The listing builds one solid part. Answer for the finished solid, in the listing's coordinates (mm). A direction names the side the tool comes from. Give positions to 0.01 mm unless a question says otherwise; leave off trailing zeros. Write each loop counter-clockwise with the first axis right and the second up, starting at its lowest first coordinate (ties: lowest second). Pieces come first, ordered by that corner, then holes. Notation, with made-up numbers: M 17,47 L 70,47 A35 ccw 70,86 Z; hole C 78,75 d3. An arc over 180 degrees is marked long. Answer as a JSON object with one key per item and string values.
```python
from build123d import *

# Parameters (mm, degrees)
SKETCH_W      = 135
SKETCH_H      = 117
SKETCH_R      = 1.75
PAD_DEPTH     = 5
SKETCH001_W   = 36
SKETCH001_H   = 19.7
PAD001_DEPTH  = 4.8
SKETCH002_W   = 6
SKETCH002_H   = 28
SKETCH002_R   = 1.5
PAD002_DEPTH  = 4
SKETCH003_W   = 6
SKETCH003_H   = 28
SKETCH003_R   = 1.5
PAD003_DEPTH  = 4
SKETCH004_W   = 6
SKETCH004_H   = 28
SKETCH004_R   = 1.5
PAD004_DEPTH  = 4
SKETCH005_W   = 6
SKETCH005_H   = 28
SKETCH005_R   = 1.5
PAD005_DEPTH  = 4
SKETCH006_R   = 2.5
SKETCH006_R_2 = 1.65
PAD006_DEPTH  = 5
SKETCH007_W   = 4
SKETCH007_H   = 20
PAD007_DEPTH  = 8
SKETCH009_W   = 6
SKETCH009_H   = 6
SKETCH009_R   = 1.5
PAD009_DEPTH  = 32
FILLET_R      = 4


with BuildPart() as part:
    # Sketch → Pad (new body)
    with BuildSketch(Plane.XY):
        Rectangle(SKETCH_W, SKETCH_H)
        with Locations((-51.402592, 19.5)):
            Circle(SKETCH_R, mode=Mode.SUBTRACT)
        with Locations((-51.402592, -19.5)):
            Circle(SKETCH_R, mode=Mode.SUBTRACT)
    extrude(amount=-PAD_DEPTH)

    # Sketch001 (on Face7 of Pad) → Pad001 (join)
    with BuildSketch(Plane.XY):
        with Locations((48.9, 43.23)):
            Rectangle(SKETCH001_W, SKETCH001_H)
        with Locations((48.9, -42.47)):
            Rectangle(SKETCH001_W, SKETCH001_H)
    extrude(amount=PAD001_DEPTH)

    # Sketch002 (on Face9 of Pad001) → Pad002 (join)
    with BuildSketch(Plane.XZ.offset(52.32)):
        with Locations((35.8, 14)):
            Rectangle(SKETCH002_W, SKETCH002_H)
        with Locations((35.92, 25.2)):
            Circle(SKETCH002_R, mode=Mode.SUBTRACT)
        with Locations((35.92, 7.2)):
            Circle(SKETCH002_R, mode=Mode.SUBTRACT)
    extrude(amount=PAD002_DEPTH)

    # Sketch003 (on Face14 of Pad002) → Pad003 (join)
    with BuildSketch(Plane(origin=(0, -32.62, 0), x_dir=(-1, 0, 0), z_dir=(0, 1, 0))):
        with Locations((-35.8, 14)):
            Rectangle(SKETCH003_W, SKETCH003_H)
        with Locations((-36, 25.2)):
            Circle(SKETCH003_R, mode=Mode.SUBTRACT)
        with Locations((-36, 7.2)):
            Circle(SKETCH003_R, mode=Mode.SUBTRACT)
    extrude(amount=PAD003_DEPTH)

    # Sketch004 (on Face22 of Pad003) → Pad004 (join)
    with BuildSketch(Plane.XZ.offset(-33.38)):
        with Locations((35.8, 14)):
            Rectangle(SKETCH004_W, SKETCH004_H)
        with Locations((36, 25.2)):
            Circle(SKETCH004_R, mode=Mode.SUBTRACT)
        with Locations((36, 7.2)):
            Circle(SKETCH004_R, mode=Mode.SUBTRACT)
    extrude(amount=PAD004_DEPTH)

    # Sketch005 (on Face27 of Pad004) → Pad005 (join)
    with BuildSketch(Plane(origin=(0, 53.08, 0), x_dir=(-1, 0, 0), z_dir=(0, 1, 0))):
        with Locations((-35.8, 14)):
            Rectangle(SKETCH005_W, SKETCH005_H)
        with Locations((-36, 25.2)):
            Circle(SKETCH005_R, mode=Mode.SUBTRACT)
        with Locations((-36, 7.2)):
            Circle(SKETCH005_R, mode=Mode.SUBTRACT)
    extrude(amount=PAD005_DEPTH)

    # Sketch006 (on Face4 of Pad005) → Pad006 (join)
    with BuildSketch(Plane.XY):
        with Locations((-11.605191, 51.606171)):
            Circle(SKETCH006_R)
        with Locations((-11.605191, 51.606171)):
            Circle(SKETCH006_R_2, mode=Mode.SUBTRACT)
        with Locations((-58.73457, 51.606171)):
            Circle(SKETCH006_R)
        with Locations((-58.73457, 51.606171)):
            Circle(SKETCH006_R_2, mode=Mode.SUBTRACT)
        with Locations((-58.73457, 28.106171)):
            Circle(SKETCH006_R)
        with Locations((-58.73457, 28.106171)):
            Circle(SKETCH006_R_2, mode=Mode.SUBTRACT)
        with Locations((-11.605191, 28.106171)):
            Circle(SKETCH006_R)
        with Locations((-11.605191, 28.106171)):
            Circle(SKETCH006_R_2, mode=Mode.SUBTRACT)
        with Locations((-19.259457, -13.335944)):
            Circle(SKETCH006_R)
        with Locations((-19.259457, -13.335944)):
            Circle(SKETCH006_R_2, mode=Mode.SUBTRACT)
        with Locations((-56.759457, -13.335944)):
            Circle(SKETCH006_R)
        with Locations((-56.759457, -13.335944)):
            Circle(SKETCH006_R_2, mode=Mode.SUBTRACT)
        with Locations((-56.759457, -50.835944)):
            Circle(SKETCH006_R)
        with Locations((-56.759457, -50.835944)):
            Circle(SKETCH006_R_2, mode=Mode.SUBTRACT)
        with Locations((-19.259457, -50.835944)):
            Circle(SKETCH006_R)
        with Locations((-19.259457, -50.835944)):
            Circle(SKETCH006_R_2, mode=Mode.SUBTRACT)
    extrude(amount=PAD006_DEPTH)

    # Sketch007 (on Face4 of Pad006) → Pad007 (join)
    with BuildSketch(Plane.XY):
        with Locations((63.12, -1.77)):
            Rectangle(SKETCH007_W, SKETCH007_H)
        with Locations((-9.38, -1.77)):
            Rectangle(SKETCH007_W, SKETCH007_H)
    extrude(amount=PAD007_DEPTH)

    # Sketch009 (on Face4 of Pad007) → Pad009 (join)
    with BuildSketch(Plane.XY):
        with Locations((-5, 48.093207)):
            Rectangle(SKETCH009_W, SKETCH009_H)
        with Locations((-5, 48.093207)):
            Circle(SKETCH009_R, mode=Mode.SUBTRACT)
        with Locations((-5, -46.319558)):
            Rectangle(SKETCH009_W, SKETCH009_H)
        with Locations((-5, -46.319558)):
            Circle(SKETCH009_R, mode=Mode.SUBTRACT)
    extrude(amount=PAD009_DEPTH)

    # Fillet
    fillet_edges = [part.edges().sort_by_distance(p)[0] for p in [
        (-67.5, -58.5, -2.5),
        (-67.5, 58.5, -2.5),
        (67.5, -58.5, -2.5),
        (67.5, 58.5, -2.5),
    ]]
    fillet(fillet_edges, radius=FILLET_R)


with BuildPart() as part_1:
    # Body placement: moved
    add(part.part.moved(Location((0, 0, -5))))


solid = part_1.part
```
1. A cutting plane is placed at D-D, the plane z = 16. Give the vertices of the cut face in (x, y).
Verdict:
{"outline": "M -8,-49.32 L -2,-49.32 L -2,-43.32 L -8,-43.32 Z; M -8,45.09 L -2,45.09 L -2,51.09 L -8,51.09 Z; M 32.8,-56.32 L 38.8,-56.32 L 38.8,-52.32 L 32.8,-52.32 Z; M 32.8,-32.62 L 38.8,-32.62 L 38.8,-28.62 L 32.8,-28.62 Z; M 32.8,29.38 L 38.8,29.38 L 38.8,33.38 L 32.8,33.38 Z; M 32.8,53.08 L 38.8,53.08 L 38.8,57.08 L 32.8,57.08 Z; hole C -5,-46.32 d3; hole C -5,48.09 d3"}
2. For faces 1 (the flat face through (36, -32.62, 12)), 2 (the flat face through (-55, -14, 0)), 3 (the cylindrical face through (-58.949, 53.242, -2.535)), 4 (the flat face through (53, 33.38, -3)), 5 (the flat face through (30.9, -43, -3)), determine the directions among +Z, -Z, +X, -X, +Y, -Y from which every point of the face is accessible in a straight line to the end or side of a thin tool.
Verdict:
{"face 1": "+Z, +X, -X", "face 2": "+Z, -X, +Y, -Y", "face 3": "+Z", "face 4": "+Z, +X", "face 5": "+Z, +Y, -Y"}
3. Consider line 1 along Y through (x, z) = (-5, 7); line 2 along Y through (x, z) = (37.5, 6); line 3 along Z through (x, y) = (36, -31.4). Determine where each line is inside the solid, lowest interval first.
Verdict:
{"line 1": "y = -49.32 to -47.82, -44.82 to -43.32, 45.09 to 46.59, 49.59 to 51.09", "line 2": "y = -56.32 to -52.32, -32.62 to -28.62, 29.38 to 33.38, 53.08 to 57.08", "line 3": "z = -10 to 0.7, 3.7 to 18.7, 21.7 to 23"}
4. Flat-ended cylindrical pins translate along their axes: pin 1 (6.5 mm diameter, centred on x = -4.5, z = 10.5, fed in from -Y); pin 2 (4.5 mm diameter, centred on x = -8.5, y = -6.5, fed in from +Z); pin 3 (4.5 mm diameter, centred on y = 31.5, z = 11, fed in from -X). Find the tip coordinate at first contact, or state that the pin passes through.
Verdict:
{"pin 1": "stops at y = -49.32", "pin 2": "stops at z = 3", "pin 3": "stops at x = 32.8"}
5. A cutting plane is placed at A-A, the plane x = -51.5. Give the vertices of the cut face in (y, z).
Verdict:
{"outline": "M -58.5,-10 L -21.25,-10 L -21.25,-5 L -58.5,-5 Z; M -17.75,-10 L 17.75,-10 L 17.75,-5 L -17.75,-5 Z; M 21.25,-10 L 58.5,-10 L 58.5,-5 L 21.25,-5 Z"}
6. The mould has two halves that part along Y. Classify faces 6 (the cylindrical face through (-58.408, -50.763, -2.535)), 7 (the flat face through (53, -52.32, -3)), 8 (the cylindrical face through (34.8, 31.4, 1.3)), 9 (the flat face through (36, -52.32, 12)): released by +Y, released by -Y, zero draft, split by the parting line, or undercut.
Verdict:
{"face 6": "undercut", "face 7": "released by -Y", "face 8": "zero draft", "face 9": "undercut"}
7. A cutting plane is placed at B-B, the plane y = 19.5. Give the vertices of the cut face in (x, z).
Verdict:
{"outline": "M -67.5,-10 L -53.15,-10 L -53.15,-5 L -67.5,-5 Z; M -49.65,-10 L 67.5,-10 L 67.5,-5 L -49.65,-5 Z"}
8. A cutting plane is placed at C-C, the plane x = 51. Give the vertices of the cut face in (y, z).
Verdict:
{"outline": "M -58.5,-10 L 58.5,-10 L 58.5,-5 L 53.08,-5 L 53.08,-0.2 L 33.38,-0.2 L 33.38,-5 L -32.62,-5 L -32.62,-0.2 L -52.32,-0.2 L -52.32,-5 L -58.5,-5 Z"}
